The listing builds one solid part. Answer for the finished solid, in the listing's coordinates (mm). A direction names the side the tool comes from. Give positions to 0.01 mm unless a question says otherwise; leave off trailing zeros. Order: outer loops, then holes, each group sorted by start corner. A loop starts at its lowest first (then second) coordinate and runs counter-clockwise, first axis right, second up. Notation, with made-up numbers: (72, 68) - (103, 68) arc R15 cw to (103, 85) - close; hole circle Ø2 at (64.25, -12). An arc over 180 degrees is marked (long way). Answer as a JSON object with one key per item and string values. Group by question number.
Q1. A cutting plane is placed at B-B, the plane x = 83. Give the vertices of the cut face in (y, z).
Q2. For faces 1 (the face through (95, 33.02, 13)), 2 (the face through (38.107, 29, 13)), determine the directions among +Z, -Z, +X, -X, +Y, -Y from which every point of the face is accessible in a straight line to the end or side of a thin tool.
Q3. Consider line 1 (Y direction, x = 135.5, z = 9.5); line 2 (X direction, y = 15, z = 13); line 3 (X direction, y = 14, z = 5.5). Determine where each line is inside the solid, lowest interval first.
Q4. A cutting plane is placed at A-A, the plane y = 12.7. Give the vertices of the cut face in (x, z), and give its area (3 significant figures).
Q5. Given pin 1 (3 mm diameter, centred on x = 137.5, z = 13, fed in from +Y); pin 2 (2.5 mm diameter, centred on y = 29, z = 15.5, fed in from -X), each flat-ended and moving along its own axis, determine where each tip first touches the part or whether it passes through.
Q6. A cutting plane is placed at C-C, the plane y = 30.5. Count the separate pieces of the cut face and the enclosed holes in it, and give its area (3 significant figures).
Q7. The mould has two halves that part along X. Classify faces 3 (the face through (99.067, 29, 13)), 4 (the face through (75, 17, 25.4)), 5 (the face through (152.4, 16, 13)): released by +X, released by -X, zero draft, split by the parting line, or undercut.
from build123d import *

# Parameters (mm, degrees)
SKETCH1_R        = 3.175
EXTRUSION2_DEPTH = 25.4


with BuildPart() as part:
    # Sketch1 → Extrusion2 (new body)
    with BuildSketch(Plane.XY):
        Polygon((0, 0), (152.4, 0), (152.4, 25.4), (152.4, 33.02), (144.767375471, 33.02), (144.767375471, 25.4), (134.626900767, 25.4), (134.626900767, 33.02), (127.006900767, 33.02), (127.006900767, 25.4), (116.846900767, 25.4), (116.846900767, 33.02), (109.226900767, 33.02), (109.226900767, 25.4), (99.066900767, 25.4), (99.066900767, 33.02), (91.446900767, 33.02), (91.446900767, 25.4), (81.286900767, 25.4), (81.286900767, 33.02), (73.666900767, 33.02), (73.666900767, 25.4), (63.506900767, 25.4), (63.506900767, 33.02), (55.886900767, 33.02), (55.886900767, 25.4), (45.726900767, 25.4), (45.726900767, 33.02), (38.106900767, 33.02), (38.106900767, 25.4), (27.946900767, 25.4), (27.946900767, 33.02), (20.326900767, 33.02), (20.326900767, 25.4), (10.166900767, 25.4), (10.166900767, 33.02), (2.546900767, 33.02), (2.546900767, 25.4), (0, 25.4), align=None)
        with Locations((12.694659047, 12.7)):
            Circle(SKETCH1_R, mode=Mode.SUBTRACT)
    extrude(amount=EXTRUSION2_DEPTH)


solid = part.part
Reply:
{
 "1": {"outline": "(0, 0) - (25.4, 0) - (25.4, 25.4) - (0, 25.4) - close"},
 "2": {"face 1": "+Z, -Z, +X, -X, +Y", "face 2": "+Z, -Z, +Y"},
 "3": {"line 1": "y = 0 to 25.4", "line 2": "x = 0 to 10.51, 14.88 to 152.4", "line 3": "x = 0 to 9.8, 15.59 to 152.4"},
 "4": {"outline": "(0, 0) - (9.52, 0) - (9.52, 25.4) - (0, 25.4) - close; (15.87, 0) - (152.4, 0) - (152.4, 25.4) - (15.87, 25.4) - close", "area": "3,710 mm^2"},
 "5": {"pin 1": "stops at y = 25.4", "pin 2": "stops at x = 2.55"},
 "6": {"separate pieces": "9", "enclosed holes": "0", "area": "1,740 mm^2"},
 "7": {"face 3": "undercut", "face 4": "zero draft", "face 5": "released by +X"}
}
